from build123d import *

# Parameters (mm, degrees)
F2_R          = 7.186555345
F3_ANGLE_BACK = 40
F3_ANGLE      = 70


with BuildPart() as f1:
    # F0 (on Front) → F1 (revolve)
    with BuildSketch(Plane.XZ):
        Polygon((0, 20), (0, 0), (150, 0), (150, 20), (115, 20), (115, 35), (90, 35), (90, 15), (60, 15), (60, 35), (35, 35), (35, 20), align=None)
    revolve(axis=Axis((75, 0, 0), (-1, 0, 0)))

    # F2 (on Front) → F3 (revolve, cut)
    with BuildSketch(Plane.XZ, mode=Mode.PRIVATE) as f3_sk:
        with Locations((47.9439608753, 34.906566143)):
            Circle(F2_R)
    revolve(f3_sk.sketch.rotate(Axis((83.0608084798, 0, 0), (-1, 0, 0)), -F3_ANGLE_BACK), axis=Axis((83.0608084798, 0, 0), (-1, 0, 0)), revolution_arc=F3_ANGLE, mode=Mode.SUBTRACT)


solid = f1.part
Could you check a few things on this model? Use its own coordinates, in mm. A direction names the side the tool comes from. Coordinates: 2 decimals unless noted, no trailing zeros. Write each loop counter-clockwise with the first axis right and the second up, starting at its lowest first coordinate (ties: lowest second). Pieces come first, ordered by that corner, then holes. Notation, with made-up numbers: (-26, -15) - (27, -15) arc R12 cw to (27, 7) - close; hole circle Ø4 at (73, 59.5). An arc over 180 degrees is marked (long way). Put each result on its own line as item: value. Start each with the question number.
Q1. I'm going to push flat-ended pins straight in: P1, Ø6, axis at x = 19.5, z = -5, coming from the -Y side; P2, Ø4, axis at y = -22.5, z = 17.5, coming from the -X side; P3, Ø6, axis at x = 81.5, y = 6.5, coming from the -Z side; P4, Ø1.5, axis at y = -25.5, z = -26, coming from the -X side. Where does each tip first touch, or does it pass through?
Q2. Please list where these lines run through material, in increasing order: L1, parallel to X at y = -26, z = -22; L2, parallel to X at y = -5, z = -16; L3, parallel to X at y = 2, z = 31.5.
Q3. I want a section at A-A on y = -27.5. Write out the boundary of the cut face in (x, z), plus the area to 3 significant figures.
Q4. Which directions (+Z, -Z, +X, -X, +Y, -Y) give clear straight access to the entire face, cutting with the end or side of a thin tool? Please do faces 4 (the cylindrical face through (74.79, 0.66, -14.985)), 5 (the flat face through (115, -15, -15)), 6 (the flat face through (47.84, -20.71, 24.68)).
Q5. I want a section at D-D on x = 120. Write out the boundary of the cut face in (y, z).
Q6. I want a section at C-C on y = 0. Write out the boundary of the cut face in (x, z).
Q7. Thinking about a two-plate mould opening in X: for faces 1 (the cylindrical face through (102, -21, -28)), 2 (the flat face through (90, -7, 15)), 3 (the flat face through (0, 0, 0)), which applies, pulls with the +X half, pulls with the -X half, needs draft (parallel to the pull), parting line crosses it, or undercut?
Q8. I want a section at B-B on z = 0. Write out the boundary of the cut face in (x, y).
Checks:
1. P1: y = -19.9
1. P2: x = 35
1. P3: z = -14.59
1. P4: through
2. L1: 35 to 60, 90 to 115
2. L2: 0 to 60, 90 to 150
2. L3: 35 to 41.58, 54.31 to 60, 90 to 115
3. outline: (35, -21.65) - (60, -21.65) - (60, 21.65) - (35, 21.65) - close; (90, -21.65) - (115, -21.65) - (115, 21.65) - (90, 21.65) - close
3. area: 2,170 mm²
4. face 4: none
4. face 5: +X
4. face 6: +Z
5. outline: circle Ø40 at (0, 0)
6. outline: (0, -20) - (35, -20) - (35, -35) - (60, -35) - (60, -15) - (90, -15) - (90, -35) - (115, -35) - (115, -20) - (150, -20) - (150, 20) - (115, 20) - (115, 35) - (90, 35) - (90, 15) - (60, 15) - (60, 35) - (55.13, 35) arc R7.19 cw (long way) to (40.76, 35) - (35, 35) - (35, 20) - (0, 20) - close
7. face 1: needs draft
7. face 2: undercut
7. face 3: pulls with the -X half
8. outline: (0, -20) - (35, -20) - (35, -35) - (60, -35) - (60, -15) - (90, -15) - (90, -35) - (115, -35) - (115, -20) - (150, -20) - (150, 20) - (115, 20) - (115, 35) - (90, 35) - (90, 15) - (60, 15) - (60, 35) - (35, 35) - (35, 20) - (0, 20) - close
